Verification items for this drawing (mm, ordinates from the low corner). A direction names the side the tool comes from. Round coordinates to 2 decimals unless told otherwise and drop trailing zeros. Loops run counter-clockwise (first coordinate to the right, second up) from the corner with the lowest first, then second, coordinate; pieces in that order, holes last. Notation, with made-up numbers: (9, 38.25) - (30, 38.25) arc R25 cw to (30, 77.25) - close; hole circle Ø8 at (0.25, -7). An arc over 180 degrees is marked (long way). Write item = value, one per line.
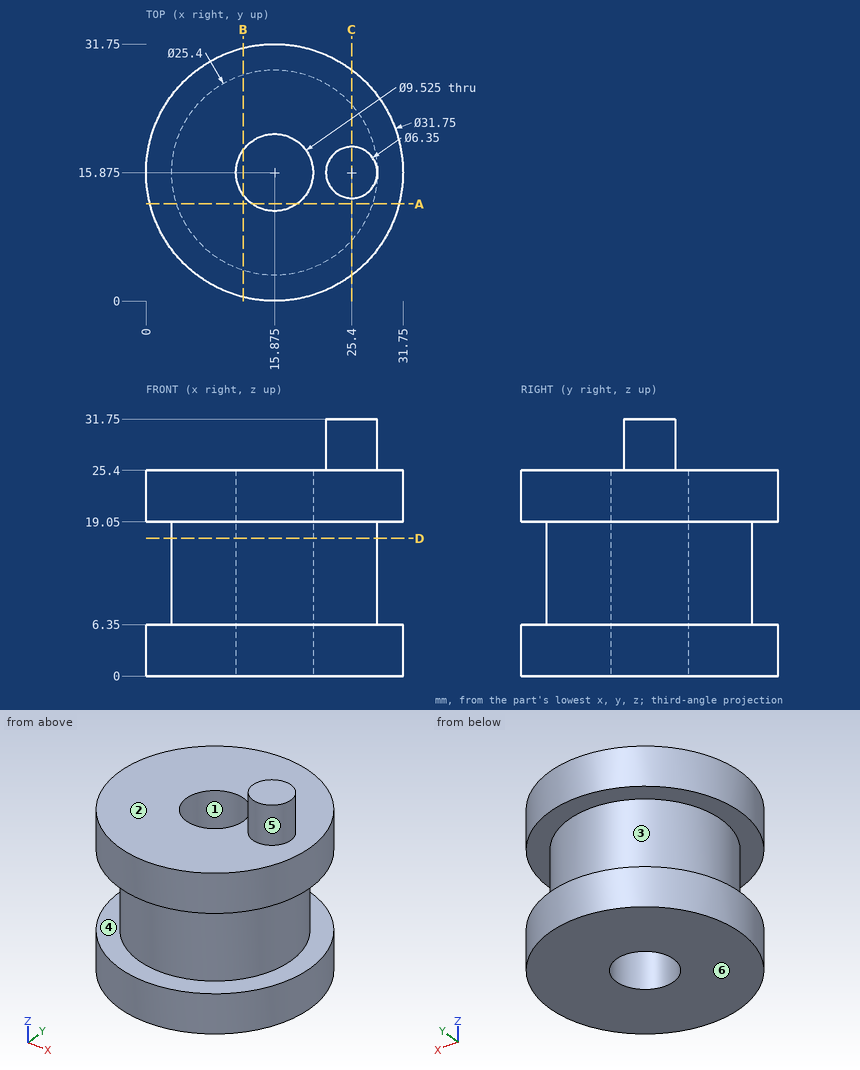
(1) Section check D-D (z = 17). Enter the section's corners in (x, y) (1 decimal).
Answers follow:
outline = circle Ø25.4 at (15.9, 15.9); hole circle Ø9.5 at (15.9, 15.9)
(2) Scan lines: L1, parallel to Z at x = 3, y = 21.5; L2, parallel to Z at x = 22.5, y = 11; L3, parallel to Y at x = 16.5, z = 17.5. Record each from-to range of solid material in increasing order. Write a range as [from, to].
Answers follow:
L1 = [0, 6.35], [19.05, 25.4]
L2 = [0, 25.4]
L3 = [3.19, 11.15], [20.6, 28.56]
(3) Gauge pin test, flat ends, axial feed: pin 1 (4 mm diameter, centred on y = 25, z = 5, fed in from +X); pin 2 (5 mm diameter, centred on x = 19.5, z = 7, fed in from +Y); pin 3 (2 mm diameter, centred on x = 18.5, y = 10.5, fed in from +Z). Record the tip position at first contact, or that the pin passes through.
Answers follow:
pin_1 = 30.06
pin_2 = 31.7
pin_3 = 25.4
(4) Section check C-C (x = 25.4). Enter the section's corners in (y, z) (3 decimals).
Answers follow:
outline = (3.175, 0) - (28.575, 0) - (28.575, 6.35) - (24.275, 6.35) - (24.275, 19.05) - (28.575, 19.05) - (28.575, 25.4) - (19.05, 25.4) - (19.05, 31.75) - (12.7, 31.75) - (12.7, 25.4) - (3.175, 25.4) - (3.175, 19.05) - (7.475, 19.05) - (7.475, 6.35) - (3.175, 6.35) - close
(5) Set-up check for the marked faces 4, 5 and 6: record each of +Z, -Z, +X, -X, +Y, -Y from which the full face is reachable in a straight line by a thin tool's end or side.
Answers follow:
face_4 = none
face_5 = +Z
face_6 = -Z, +X, -X, +Y, -Y
(6) Section check A-A (y = 12). Enter the section's corners in (x, z).
Answers follow:
outline = (0.48, 0) - (13.11, 0) - (13.11, 25.4) - (0.48, 25.4) - (0.48, 19.05) - (3.78, 19.05) - (3.78, 6.35) - (0.48, 6.35) - close; (18.64, 0) - (31.27, 0) - (31.27, 6.35) - (27.97, 6.35) - (27.97, 19.05) - (31.27, 19.05) - (31.27, 25.4) - (18.64, 25.4) - close
(7) Mould release check, pull along Z, two halves, no side actions. Record for the marked faces 1, 2 and 3: pulls with the +Z half, pulls with the -Z half, needs draft (parallel to the pull), parting line crosses it, or undercut.
Answers follow:
face_1 = needs draft
face_2 = pulls with the +Z half
face_3 = undercut
